CAD build for the part. Positions are in the model's coordinates, mm. A direction names the side the tool comes from. Round coordinates to 2 decimals unless told otherwise and drop trailing zeros. Write each loop counter-clockwise with the first axis right and the second up, starting at its lowest first coordinate (ties: lowest second). Pieces come first, ordered by that corner, then holes. Notation, with made-up numbers: (3, -6) - (53, -6) arc R20 ccw to (53, 14) - close; hole circle Ø8 at (67.25, 28). An arc over 180 degrees is marked (long way). Put each result on its own line as item: value. Start each with the question number.
Item 1: Cut at B-B (z = 2.25). Give the cut face in (x, y).
Item 2: Cut at C-C (x = 4). Give the cut face in (y, z), and give its area (3 significant figures).
Item 3: Cut at D-D (y = 12.5). Give the cut face in (x, z).
Item 4: Pin check, flat tips, straight feed: pin 1 Ø10 at (x, y) = (16, 4.5) entering from +Z; pin 2 Ø3 at (y, z) = (36, 10) entering from -X; pin 3 Ø3 at (y, z) = (4, 15.5) entering from +X. Stop position of each tip, or through.
Item 5: 3-axis set-ups, long thin cutter, end or side, ignore diameter. For faces 1 (the flat face through (6, 3, 12)), 2 (the flat face through (38, 6, 3)), 3 (the cylindrical face through (0, 20, 12)), 4 (the flat face through (0, 20, 1)), 5 (the cylindrical face through (39.1, 39.14, 1.52)): which of +Z, -Z, +X, -X, +Y, -Y reach the whole face in a straight line?
Item 6: Mould opens along X. For faces 6 (the cylindrical face through (0.86, 39.1, 1.52)), 7 (the cylindrical face through (40, 20, 12)), 8 (the cylindrical face through (2.85, 3.12, 1.48)) say: released by +X, released by -X, zero draft, split by the parting line, or undercut.
Item 7: Cut at A-A (z = 16). Give the cut face in (x, y), and give its area (3 significant figures).
Item 8: Drill centre lines: line 1 (Y direction, x = 4, z = 1.15); line 2 (X direction, y = 20, z = 15.75); line 3 (X direction, y = 36.25, z = 16). Where is each one in solid material? Low to high. Write a range as from..to.
```python
from build123d import *

# Parameters (mm, degrees)
CYLINDER002_R          = 12.45
CYLINDER002_DEPTH      = 55
CYLINDER002_ROLL_ANGLE = 90
CYLINDER005_R          = 18
CYLINDER005_DEPTH      = 39
BOX001_W               = 28
BOX001_H               = 8
BOX001_DEPTH           = 21
BOX001001_W            = 28
BOX001001_H            = 8
BOX001001_DEPTH        = 21
CYLINDER001_R          = 18
CYLINDER001_DEPTH      = 10
CYLINDER_R             = 1.45
CYLINDER_DEPTH         = 10
ARRAY_X_COUNT          = 2
ARRAY_X_PITCH          = 32
ARRAY_Y_COUNT          = 2
ARRAY_Y_PITCH          = 32
BOX_W                  = 40
BOX_H                  = 40
BOX_DEPTH              = 3
FILLET_R               = 3
CYLINDER004_R          = 18
CYLINDER004_DEPTH      = 21
CYLINDER003_R          = 20
CYLINDER003_DEPTH      = 21


with BuildPart() as cylinder002:
    # Cylinder002 → Cylinder002 (new body)
    with BuildSketch(Plane.XY):
        Circle(CYLINDER002_R)
    extrude(amount=CYLINDER002_DEPTH)


with BuildPart() as cylinder002_1:
    # Cylinder002 roll: moved
    add(cylinder002.part.rotate(Axis((0, 0, 0), (1, 0, 0)), CYLINDER002_ROLL_ANGLE))


with BuildPart() as cylinder002_2:
    # Cylinder002 placement: moved
    add(cylinder002_1.part.moved(Location((20, 45.000004, 16))))


with BuildPart() as cylinder005:
    # Cylinder005 → Cylinder005 (new body)
    with BuildSketch(Plane(origin=(20, 20, -6), x_dir=(1, 0, 0), z_dir=(0, 0, 1))):
        Circle(CYLINDER005_R)
    extrude(amount=CYLINDER005_DEPTH)


with BuildPart() as box001:
    # Box001 → Box001 (new body)
    with BuildSketch(Plane(origin=(6, 0, 0), x_dir=(1, 0, 0), z_dir=(0, 0, 1))):
        with Locations((14, 4)):
            Rectangle(BOX001_W, BOX001_H)
    extrude(amount=BOX001_DEPTH)


with BuildPart() as cut005:
    # Box001001 → Box001001 (new body)
    with BuildSketch(Plane(origin=(6, 32, 0), x_dir=(1, 0, 0), z_dir=(0, 0, 1))):
        with Locations((14, 4)):
            Rectangle(BOX001001_W, BOX001001_H)
    extrude(amount=BOX001001_DEPTH)

    # Fusion001: union Box001
    add(box001.part)

    # Cut004: cut Cylinder005
    add(cylinder005.part, mode=Mode.SUBTRACT)

    # Cut005: cut Cylinder002
    add(cylinder002_2.part, mode=Mode.SUBTRACT)


with BuildPart() as cylinder001:
    # Cylinder001 → Cylinder001 (new body)
    with BuildSketch(Plane(origin=(20, 20, 0), x_dir=(1, 0, 0), z_dir=(0, 0, 1))):
        Circle(CYLINDER001_R)
    extrude(amount=CYLINDER001_DEPTH)


with BuildPart() as array:
    # Cylinder → Cylinder (new body)
    with BuildSketch(Plane.XY):
        Circle(CYLINDER_R)
    extrude(amount=CYLINDER_DEPTH)

    # Array X: Array ×2


with BuildPart() as array_1:
    add(array.part)
    with Locations(*[(i * ARRAY_X_PITCH, 0, 0) for i in range(1, ARRAY_X_COUNT)]):
        add(array.part)

    # Array Y: Array ×2


with BuildPart() as array_2:
    add(array_1.part)
    with Locations(*[(0, i * ARRAY_Y_PITCH, 0) for i in range(1, ARRAY_Y_COUNT)]):
        add(array_1.part)


with BuildPart() as array_3:
    # Array placement: moved
    add(array_2.part.moved(Location((4, 4, 0))))


with BuildPart() as fillet_body:
    # Box → Box (new body)
    with BuildSketch(Plane.XY):
        with Locations((20, 20)):
            Rectangle(BOX_W, BOX_H)
    extrude(amount=BOX_DEPTH)

    # Cut: cut Array
    add(array_3.part, mode=Mode.SUBTRACT)

    # Cut001: cut Cylinder001
    add(cylinder001.part, mode=Mode.SUBTRACT)

    # Fillet
    fillet_edges = [fillet_body.edges().sort_by_distance(p)[0] for p in [
        (0, 0, 1.5),
        (0, 40, 1.5),
        (40, 0, 1.5),
        (40, 40, 1.5),
    ]]
    fillet(fillet_edges, radius=FILLET_R)


with BuildPart() as cylinder004:
    # Cylinder004 → Cylinder004 (new body)
    with BuildSketch(Plane(origin=(20, 20, 0), x_dir=(1, 0, 0), z_dir=(0, 0, 1))):
        Circle(CYLINDER004_R)
    extrude(amount=CYLINDER004_DEPTH)


with BuildPart() as fusion002:
    # Cylinder003 → Cylinder003 (new body)
    with BuildSketch(Plane(origin=(20, 20, 0), x_dir=(1, 0, 0), z_dir=(0, 0, 1))):
        Circle(CYLINDER003_R)
    extrude(amount=CYLINDER003_DEPTH)

    # Cut002: cut Cylinder004
    add(cylinder004.part, mode=Mode.SUBTRACT)

    # Fusion: union Fillet body
    add(fillet_body.part)

    # Cut003: cut Cylinder002
    add(cylinder002_2.part, mode=Mode.SUBTRACT)

    # Fusion002: union Cut005
    add(cut005.part)


solid = fusion002.part
```
Output values:
1. outline: (0, 3) arc R3 ccw to (3, 0) - (37, 0) arc R3 ccw to (40, 3) - (40, 37) arc R3 ccw to (37, 40) - (3, 40) arc R3 ccw to (0, 37) - close; hole circle Ø36 at (20, 20); hole circle Ø2.9 at (4, 4); hole circle Ø2.9 at (4, 36); hole circle Ø2.9 at (36, 4); hole circle Ø2.9 at (36, 36)
2. outline: (0, 0) - (2.55, 0) - (2.55, 3) - (0, 3) - close; (5.45, 0) - (11.75, 0) - (11.75, 21) - (8, 21) - (8, 3) - (5.45, 3) - close; (28.25, 0) - (34.55, 0) - (34.55, 3) - (32, 3) - (32, 21) - (28.25, 21) - close; (37.45, 0) - (40, 0) - (40, 3) - (37.45, 3) - close
2. area: 188 mm2
3. outline: (0, 0) - (3.64, 0) - (3.64, 21) - (1.46, 21) - (1.46, 3) - (0, 3) - close; (36.36, 0) - (40, 0) - (40, 3) - (38.54, 3) - (38.54, 21) - (36.36, 21) - close
4. pin 1: z = 7.4
4. pin 2: x = 6
4. pin 3: x = 34
5. face 1: +Z, -X, -Y
5. face 2: +Z, +X, -Y
5. face 3: +Z, -X
5. face 4: +Z, -Z, -X, +Y, -Y
5. face 5: +Z, -Z, +X, +Y
6. face 6: released by -X
6. face 7: released by +X
6. face 8: undercut
7. outline: (6, 0) - (7.55, 0) - (7.55, 7) arc R18 cw to (7.55, 33) - (7.55, 40) - (6, 40) - (6, 34.28) arc R20 ccw to (6, 5.72) - close; (32.45, 0) - (34, 0) - (34, 5.72) arc R20 ccw to (34, 34.28) - (34, 40) - (32.45, 40) - (32.45, 33) arc R18 cw to (32.45, 7) - close
7. area: 161 mm2
8. line 1: 0..2.55, 5.45..11.75, 28.25..34.55, 37.45..40
8. line 2: 0..2, 38..40
8. line 3: 6..7.55, 32.45..34
